Part model, mm, in its own coordinate system. A direction names the side the tool comes from. Coordinates: 2 decimals unless noted, no trailing zeros. Order: outer loops, then holes, each group sorted by start corner. A loop starts at its lowest first (then second) coordinate and runs counter-clockwise, first axis right, second up. Notation, with made-up numbers: M 10,-38.75 L 28,-38.75 A23 ccw 28,-14.75 Z; hole C 79.25,66 d6. An arc over 180 degrees is marked long. Answer in a Markdown table with one row per item. Add a question column.
Autodesk Inventor part; units mm, degrees
ref_plane "YZ Plane" through (0, 0, 0) normal (1, 0, 0) x (0, 1, 0)
ref_plane "XZ Plane" through (0, 0, 0) normal (0, 1, 0) x (-1, 0, 0)
ref_plane "XY Plane" through (0, 0, 0) normal (0, 0, 1) x (1, 0, 0)
sketch "スケッチ1" plane through (0, 0, 0) normal (0, 0, 1) x (1, 0, 0)
  line L0 (0, 0) -> (14.385, 0)
  line L1 (14.385, 0) -> (14.385, 22.14)
  line L2 (14.385, 22.14) -> (23.9245, 25.0353)
  line L3 (23.9245, 31.0447) -> (14.2486, 33.9814)
  line L4 (0, 0) -> (0, 43.38) construction
  arc A0 (14.2486, 33.9814) -> (0, 43.38) centre (0, 27.88) ccw
  circle A1 centre (0, 28.04) radius 4 construction
  line L5 (0, 28.04) -> (33.824, 28.04) construction
  circle A2 centre (16.215, 28.04) radius 1.5
  circle A3 centre (23.0125, 28.04) radius 1.39
  arc A4 (23.9245, 25.0353) -> (23.9245, 31.0447) centre (23.0125, 28.04) ccw
  line L6 (0, 0) -> (-14.385, 0)
  line L7 (-14.385, 0) -> (-14.385, 22.14)
  line L8 (-14.385, 22.14) -> (-23.9245, 25.0353)
  line L9 (-23.9245, 31.0447) -> (-14.2486, 33.9814)
  arc A5 (0, 43.38) -> (-14.2486, 33.9814) centre (0, 27.88) ccw
  circle A6 centre (-16.215, 28.04) radius 1.5
  circle A7 centre (-23.0125, 28.04) radius 1.39
  arc A8 (-23.9245, 31.0447) -> (-23.9245, 25.0353) centre (-23.0125, 28.04) ccw
  dimension "d0" = 15.5
  dimension "d1" = 43.38
  dimension "d2" = 15.34
  dimension "d3" = 8
  dimension "d4" = 14.385
  dimension "d5" = 5.9
  dimension "d6" = 2.78
  dimension "d7" = 3
  dimension "d8" = 16.215
  dimension "d9" = 23.0125
  dimension "d12" = 3.14
extrude "押し出し1" add sketch "スケッチ1" along normal blind 2.5
sketch "スケッチ4" plane through (0, 0, 2.5) normal (0, 0, 1) x (1, 0, 0)
  line L0 (-14.385, 0) -> (14.385, 0)
  line L1 (-14.385, 0) -> (14.385, 0)
  line L2 (14.385, 0) -> (14.385, 33.6525)
  arc A0 (14.2486, 33.9814) -> (-14.2486, 33.9814) centre (0, 27.88) ccw
  arc A1 (14.385, 33.6525) -> (-14.385, 33.6525) centre (0, 27.88) ccw
  line L3 (-14.385, 0) -> (-14.385, 33.6525)
  point P0 (0, 0)
extrude "押し出し3" add sketch "スケッチ4" along normal blind 6.5
sketch "スケッチ5" plane through (0, 0, 9) normal (0, 0, 1) x (1, 0, 0)
  line L0 (0, 0) -> (0, 28.04) construction
  circle A0 centre (0, 28.04) radius 4
  arc A1 (14.2486, 33.9814) -> (-14.2486, 33.9814) centre (0, 27.88) ccw construction
  point P0 (0, 43.38)
  dimension "d20" = 15.34
  dimension "d21" = 8
extrude "押し出し4" cut sketch "スケッチ5" against normal up to next
chamfer "面取り1" distance 0.5 angle 45 5 edges at (-14.385, 16.8263, 9) (0, 0, 9) (14.385, 16.8263, 9) (0, 43.38, 9) (-4, 28.04, 9)
properties part number "AMT102-1"
(1) Slice it at D-D (y = 20). List the corners of the cut face in (x, z) (3 decimals).
(2) Drop flat-ended pins along their axis: P1, Ø1, axis at x = -13, y = 10, coming from the -Z side; P2, Ø1, axis at x = 14, z = 1.5, coming from the +Y side; P3, Ø4, axis at y = 11.5, z = 2, coming from the +X side (3 decimals); P4, Ø2.5, axis at y = 22, z = 6, coming from the -X side (3 decimals). Give the stop position or say it passes through.
(3) Pull direction X, two halves, no side cores. Call faces 5 (the cylindrical face through (21.99, 27.1, 1.23)), 6 (the flat face through (-19.154, 32.492, 1.232)), 7 (the flat face through (19.09, 23.57, 1.23)): pulls with the +X half, pulls with the -X half, needs draft (parallel to the pull), parting line crosses it, or undercut.
(4) 3-axis set-ups, long thin cutter, end or side, ignore diameter. For faces 1 (the cylindrical face through (-23.19, 26.66, 1.23)), 2 (the flat face through (14.385, 17, 4)), 3 (the flat face through (19, 28, 2.5)), 4 (the flat face through (-14.385, 17, 4)): which of +Z, -Z, +X, -X, +Y, -Y reach the whole face in a straight line?
(5) Wall check: line 1 (X direction, y = 28, z = 3) (3 decimals); line 2 (X direction, y = 3, z = 6) (3 decimals); line 3 (X direction, y = 30, z = 1.5). Give the ranges that are in metal, low to high.
(6) Slice it at C-C (z = 1). List the corners of the cut face in (x, y) (1 decimal), and give its area (3 significant figures).
(7) Slice it at A-A (y = 28.04). State how many separate pieces and enclosed holes the cut face has, and give its area (3 significant figures).
Computed:
| question | item | result |
|---|---|---|
| 1 | outline | M -14.385,0 L 14.385,0 L 14.385,8.5 L 13.885,9 L -13.885,9 L -14.385,8.5 Z |
| 2 | P1 | stops at z = 0 |
| 2 | P2 | stops at y = 35.5 |
| 2 | P3 | stops at x = 14.385 |
| 2 | P4 | stops at x = -14.385 |
| 3 | face 5 | undercut |
| 3 | face 6 | pulls with the -X half |
| 3 | face 7 | pulls with the +X half |
| 4 | face 1 | +Z, -Z |
| 4 | face 2 | +Z, +X, -Y |
| 4 | face 3 | +Z, +X, +Y, -Y |
| 4 | face 4 | +Z, -X, -Y |
| 5 | line 1 | x = -14.385 to -4, 4 to 14.385 |
| 5 | line 2 | x = -14.385 to 14.385 |
| 5 | line 3 | x = -25.47 to -3.49, 3.49 to 25.47 |
| 6 | outline | M -23.9,25 L -14.4,22.1 L -14.4,0 L 14.4,0 L 14.4,22.1 L 23.9,25 A3.1 ccw 23.9,31 L 14.2,34 A15.5 ccw 0,43.4 A15.5 ccw -14.2,34 L -23.9,31 A3.1 ccw Z; hole C -23,28 d2.8; hole C -16.2,28 d3; hole C 0,28 d8; hole C 16.2,28 d3; hole C 23,28 d2.8 |
| 6 | area | 1,280 mm^2 |
| 7 | separate pieces | 6 |
| 7 | enclosed holes | 0 |
| 7 | area | 216 mm^2 |
